The listing builds one solid part. Answer for the finished solid, in the listing's coordinates (mm). Face numbers are marked on the shaded views. Give positions to 0.01 mm unless a question says otherwise; leave off trailing zeros. Write each loop counter-clockwise with the first axis right and the second up, starting at its lowest first coordinate (ties: lowest second). Pieces come first, ordered by that corner, then holes. Notation, with made-up numbers: (47.25, -8.75) - (94.25, -8.75) arc R18 cw to (94.25, 6.25) - close; hole circle Ø7 at (-36.5, -26.5). An arc over 180 degrees is marked (long way). Write each question's results on one line, items separated by ' | '. Start each with the question number.
Q1. Find the intervals of material crossed by probe 1 along X at (y, z) = (1, -84); probe 2 along X at (y, z) = (1.15, -16); probe 3 along X at (y, z) = (1.65, -45.5), in increasing order.
Q2. For a pull along Y with two mould halves and no side action, classify the marked faces 1 and 2 as pulls with the +Y half, pulls with the -Y half, needs draft (parallel to the pull), parting line crosses it, or undercut.
Q3. Flat-ended cylindrical pins translate along their axes: pin 1 Ø1 at (x, y) = (6, 1) entering from -Z; pin 2 Ø1 at (y, z) = (1.5, 1) entering from +X; pin 3 Ø1.5 at (x, y) = (-38, 2) entering from +Z. Find the tip coordinate at first contact, or state that the pin passes through.
Q4. Section A-A (z = -60) is taken. Determine the outline of the cut face in (x, y) (3 decimals), plus the area to 3 significant figures.
Q5. Section C-C (x = -38) is taken. Determine the outline of the cut face in (y, z) (3 decimals).
Q6. Section D-D (x = -54) is taken. Determine the outline of the cut face in (y, z) (3 decimals).
Q7. Section B-B (y = 1.5) is taken. State how many separate pieces and enclosed holes the cut face has, plus the area to 3 significant figures.
```python
from build123d import *

# Parameters (mm, degrees)
SKETCH1_R           = 2.15
SKETCH1_R_2         = 3
SKETCH1_R_3         = 1.6
SKETCH1_W           = 6.35
SKETCH1_H           = 6.35
BOSS_EXTRUDE1_DEPTH = 3.175
FILLET1_R           = 10


with BuildPart() as part:
    # Sketch1 → Boss-Extrude1 (new body)
    with BuildSketch(Plane(origin=(0, 0, 0), x_dir=(1, 0, 0), z_dir=(0, 1, 0))):
        with BuildLine():
            Line((-69.108920632, 87.491689248), (-22.994598309, -10.789274703))
            ThreePointArc((-22.994598309, -10.789274703), (0, -25.4), (22.994598309, -10.789274703))
            Line((22.994598309, -10.789274703), (69.108920632, 87.491689248))
            Line((69.108920632, 87.491689248), (40.365672746, 100.978282626))
            Line((40.365672746, 100.978282626), (0, 14.949104962))
            Line((0, 14.949104962), (-40.365672746, 100.978282626))
            Line((-40.365672746, 100.978282626), (-69.108920632, 87.491689248))
        make_face()
        with Locations((47.994, 79.863361994)):
            Circle(SKETCH1_R, mode=Mode.SUBTRACT)
        with Locations((-47.994, 79.863361994)):
            Circle(SKETCH1_R, mode=Mode.SUBTRACT)
        with Locations((-33.126889189, 48.177891883)):
            Circle(SKETCH1_R_2, mode=Mode.SUBTRACT)
        with Locations((-32.297900068, 25.811951773)):
            Circle(SKETCH1_R_3, mode=Mode.SUBTRACT)
        with Locations((-16.455165013, 33.245507178)):
            Circle(SKETCH1_R_3, mode=Mode.SUBTRACT)
        Rectangle(SKETCH1_W, SKETCH1_H, mode=Mode.SUBTRACT)
    extrude(amount=BOSS_EXTRUDE1_DEPTH)

    # Fillet1
    fillet1_edges = [part.edges().sort_by_distance(p)[0] for p in [
        (-40.365672746, 1.5875, -100.978282626),
        (40.365672746, 1.5875, -100.978282626),
        (69.108920632, 1.5875, -87.491689248),
        (-69.108920632, 1.5875, -87.491689248),
    ]]
    fillet(fillet1_edges, radius=FILLET1_R)


solid = part.part
```
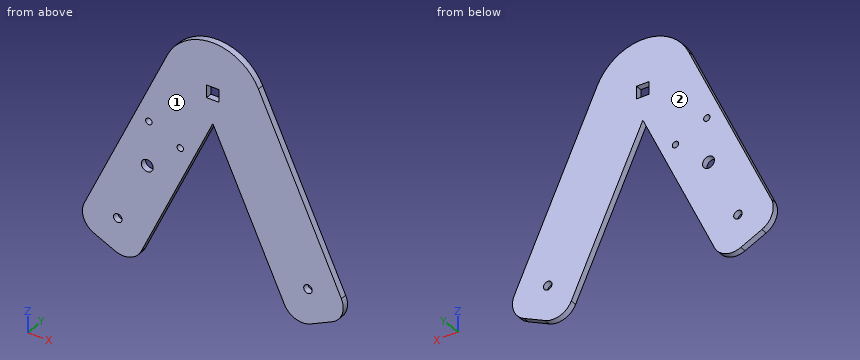
Answers below:
1) probe 1: x = -65.72 to -32.4, 32.4 to 65.72 | probe 2: x = -35.56 to -0.49, 0.49 to 35.56 | probe 3: x = -49.41 to -34.48, -31.77 to -14.33, 14.33 to 49.41
2) face 1: pulls with the -Y half | face 2: pulls with the +Y half
3) pin 1: stops at z = -28.8 | pin 2: stops at x = 27.82 | pin 3: stops at z = -19.59
4) outline: (-56.21, 0) - (-21.138, 0) - (-21.138, 3.175) - (-56.21, 3.175) - close; (21.138, 0) - (56.21, 0) - (56.21, 3.175) - (21.138, 3.175) - close | area: 223 mm2
5) outline: (0, -94.647) - (3.175, -94.647) - (3.175, -21.191) - (0, -21.191) - close
6) outline: (0, -94.581) - (3.175, -94.581) - (3.175, -55.291) - (0, -55.291) - close
7) separate pieces: 1 | enclosed holes: 6 | area: 7,340 mm2
